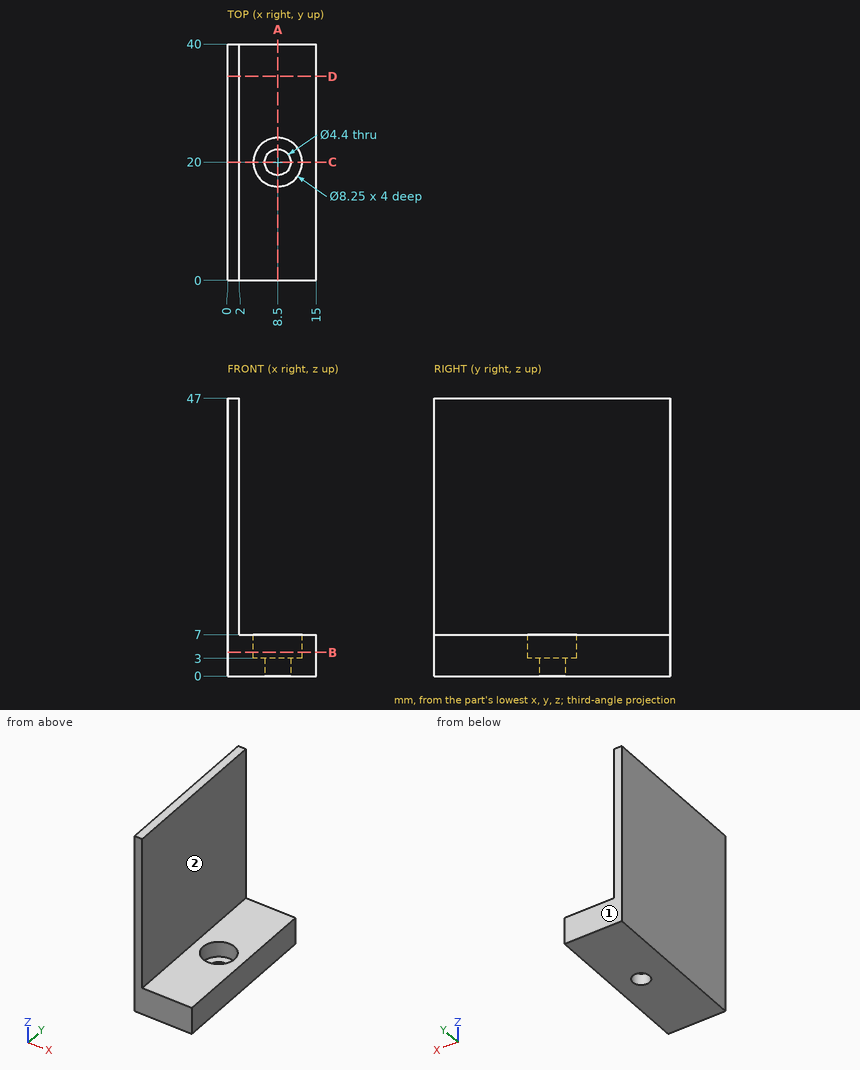
Geometry check sheet. Reference: drawing and pictorial views, mm from the part's lowest x, y, z. A direction names the side the tool comes from. Coordinates: 2 decimals unless noted, no trailing zeros. Order: outer loops, then holes, each group sorted by start corner. A loop starts at its lowest first (then second) coordinate and runs counter-clockwise, first axis right, second up. Notation, with made-up numbers: (-18.75, 49) -> (-12.75, 49) arc R16 cw to (-12.75, 70) -> close; hole circle Ø10 at (-33, 20). An arc over 180 degrees is marked (long way). Put each result on its own line as item: value. Start each with the question number.
1) Tool access check on the marked faces 1 and 2. Record the directions out of +Z, -Z, +X, -X, +Y, -Y that give a thin tool (end or side, any length) a straight path to the whole face; none if there is none.
2) Cross-section at A-A (x = 8.5). Enter the section's corners in (y, z) (3 decimals), plus the area to 3 significant figures.
3) Cross-section at C-C (y = 20). Enter the section's corners in (x, z) (3 decimals).
4) Material ranges on L1, parallel to Y at x = 8.5, z = 1.95; L2, parallel to Y at x = 8.5, z = 4.95 (3 decimals); L3, parallel to X at y = 37.5, z = 15, recorded low to high.
5) Cross-section at D-D (y = 34.5). Enter the section's corners in (x, z).
6) Cross-section at B-B (z = 4). Enter the section's corners in (x, y) (3 decimals), plus the area to 3 significant figures.
7) Go/stop test with flat-tipped pins: pin 1 (6.5 mm diameter, centred on x = 5.5, y = 26.5, fed in from +Z); pin 2 (6 mm diameter, centred on x = 6, z = 29.5, fed in from -Y); pin 3 (20 mm diameter, centred on y = 14, z = 31, fed in from +X). Record where each tip stops, or that it passes through.
Geometry check:
1. face 1: +Z, -Z, +X, -X, +Y
1. face 2: +Z, +X, +Y, -Y
2. outline: (0, 0) -> (17.8, 0) -> (17.8, 3) -> (15.875, 3) -> (15.875, 7) -> (0, 7) -> close; (22.2, 0) -> (40, 0) -> (40, 7) -> (24.125, 7) -> (24.125, 3) -> (22.2, 3) -> close
2. area: 234 mm^2
3. outline: (0, 0) -> (6.3, 0) -> (6.3, 3) -> (4.375, 3) -> (4.375, 7) -> (2, 7) -> (2, 47) -> (0, 47) -> close; (10.7, 0) -> (15, 0) -> (15, 7) -> (12.625, 7) -> (12.625, 3) -> (10.7, 3) -> close
4. L1: y = 0 to 17.8, 22.2 to 40
4. L2: y = 0 to 15.875, 24.125 to 40
4. L3: x = 0 to 2
5. outline: (0, 0) -> (15, 0) -> (15, 7) -> (2, 7) -> (2, 47) -> (0, 47) -> close
6. outline: (0, 0) -> (15, 0) -> (15, 40) -> (0, 40) -> close; hole circle Ø8.25 at (8.5, 20)
6. area: 547 mm^2
7. pin 1: stops at z = 7
7. pin 2: passes through
7. pin 3: stops at x = 2
